from build123d import *

# Parameters (mm, degrees)
SKETCH7_W           = 90
SKETCH7_H           = 65
BOSS_EXTRUDE2_DEPTH = 65
SKETCH10_W          = 86
SKETCH10_H          = 61
CUT_EXTRUDE2_DEPTH  = 62
SKETCH12_R          = 15
CUT_EXTRUDE3_DEPTH  = 91
SKETCH13_R          = 21
SKETCH13_R_2        = 3
CUT_EXTRUDE4_DEPTH  = 2
SKETCH14_W          = 7
SKETCH14_H          = 17.962946586
CUT_EXTRUDE5_DEPTH  = 5
SKETCH15_W          = 84
SKETCH15_H          = 26.21557427
CUT_EXTRUDE6_DEPTH  = 5
SKETCH17_W          = 30
SKETCH17_H          = 32.5
BOSS_EXTRUDE3_DEPTH = 15
SKETCH18_W          = 12.726486876
SKETCH18_H          = 30.948281703
CUT_EXTRUDE7_DEPTH  = 91
SKETCH20_W          = 24.28117476
SKETCH20_H          = 6.721130416
BOSS_EXTRUDE4_DEPTH = 10
SKETCH21_W          = 21.308601662
SKETCH21_H          = 6.528068718
CUT_EXTRUDE9_DEPTH  = 52.082060801
BOSS_EXTRUDE5_DEPTH = 5
SKETCH24_R          = 1.516132664
SKETCH24_R_2        = 1.46792115
CUT_EXTRUDE10_DEPTH = 3
SKETCH25_R          = 2.5
CUT_EXTRUDE11_DEPTH = 1


with BuildPart() as part:
    # Sketch7 → Boss-Extrude2 (new body)
    with BuildSketch(Plane(origin=(0, 0, 0), x_dir=(1, 0, 0), z_dir=(0, 1, 0))):
        Rectangle(SKETCH7_W, SKETCH7_H)
    extrude(amount=-BOSS_EXTRUDE2_DEPTH)

    # Sketch10 → Cut-Extrude2 (cut)
    with BuildSketch(Plane(origin=(0, 0, 0), x_dir=(1, 0, 0), z_dir=(0, 1, 0))):
        Rectangle(SKETCH10_W, SKETCH10_H)
    extrude(amount=-CUT_EXTRUDE2_DEPTH, mode=Mode.SUBTRACT)

    # Sketch12 → Cut-Extrude3 (cut, through all)
    with BuildSketch(Plane.ZY.offset(45)):
        with Locations((0, -32.5)):
            Circle(SKETCH12_R)
    extrude(amount=-CUT_EXTRUDE3_DEPTH, mode=Mode.SUBTRACT)

    # Sketch13 → Cut-Extrude4 (cut)
    with BuildSketch(Plane.XY.offset(32.5)):
        with Locations((0, -32.5)):
            Circle(SKETCH13_R)
        with Locations((-38.356194479, -9.309094371)):
            Circle(SKETCH13_R_2)
        with Locations((-38.356194479, -19.309094371)):
            Circle(SKETCH13_R_2)
        with Locations((-38.356194479, -29.309094371)):
            Circle(SKETCH13_R_2)
        with Locations((-38.356194479, -39.309094371)):
            Circle(SKETCH13_R_2)
        with Locations((36.896991428, -19.309094371)):
            Circle(SKETCH13_R_2)
        with Locations((36.896991428, -29.309094371)):
            Circle(SKETCH13_R_2)
    extrude(amount=-CUT_EXTRUDE4_DEPTH, mode=Mode.SUBTRACT)

    # Sketch14 → Cut-Extrude5 (cut)
    with BuildSketch(Plane(origin=(45, 0, 0), x_dir=(0, 0, -1), z_dir=(1, 0, 0))):
        with Locations((26, -52.018526707)):
            Rectangle(SKETCH14_W, SKETCH14_H)
    extrude(amount=-CUT_EXTRUDE5_DEPTH, mode=Mode.SUBTRACT)

    # Sketch15 → Cut-Extrude6 (cut)
    with BuildSketch(Plane.XZ.offset(65)):
        with Locations((0, -13.392212865)):
            Rectangle(SKETCH15_W, SKETCH15_H)
    extrude(amount=-CUT_EXTRUDE6_DEPTH, mode=Mode.SUBTRACT)

    # Sketch17 → Boss-Extrude3 (add)
    with BuildSketch(Plane(origin=(0, 0, -32.5), x_dir=(-1, 0, 0), z_dir=(0, 0, -1))):
        with Locations((-30, -16.25)):
            Rectangle(SKETCH17_W, SKETCH17_H)
        with Locations((30, -16.25)):
            Rectangle(SKETCH17_W, SKETCH17_H)
    extrude(amount=BOSS_EXTRUDE3_DEPTH)

    # Sketch18 → Cut-Extrude7 (cut, through all)
    with BuildSketch(Plane(origin=(45, 0, 0), x_dir=(0, 0, -1), z_dir=(1, 0, 0))):
        with Locations((40.003797932, -17.025859149)):
            Rectangle(SKETCH18_W, SKETCH18_H)
    extrude(amount=-CUT_EXTRUDE7_DEPTH, mode=Mode.SUBTRACT)

    # Sketch20 → Boss-Extrude4 (add)
    with BuildSketch(Plane(origin=(0, 0, -32.5), x_dir=(-1, 0, 0), z_dir=(0, 0, -1))):
        with Locations((0, -57.278504407)):
            Rectangle(SKETCH20_W, SKETCH20_H)
        with Locations((0, -17.278504407)):
            Rectangle(SKETCH20_W, SKETCH20_H)
    extrude(amount=BOSS_EXTRUDE4_DEPTH)

    # Sketch21 → Cut-Extrude9 (cut, through all)
    with BuildSketch(Plane(origin=(0, -13.917939199, 0), x_dir=(1, 0, 0), z_dir=(0, 1, 0))):
        with Locations((-0.070940944, 37.501061987)):
            Rectangle(SKETCH21_W, SKETCH21_H)
    extrude(amount=-CUT_EXTRUDE9_DEPTH, mode=Mode.SUBTRACT)

    # Sketch23 → Boss-Extrude5 (add)
    with BuildSketch(Plane(origin=(0, 0, 0), x_dir=(1, 0, 0), z_dir=(0, 1, 0))):
        with BuildLine():
            Line((43, -28.521055724), (43, -30.5))
            Line((43, -30.5), (41.021055724, -30.5))
            ThreePointArc((41.021055724, -30.5), (41.600675083, -29.100675083), (43, -28.521055724))
        make_face()
        with BuildLine():
            Line((-43, -28.521055724), (-43, -30.5))
            Line((-43, -30.5), (-41.021055724, -30.5))
            ThreePointArc((-41.021055724, -30.5), (-41.600675083, -29.100675083), (-43, -28.521055724))
        make_face()
    extrude(amount=-BOSS_EXTRUDE5_DEPTH)

    # Sketch24 → Cut-Extrude10 (cut)
    with BuildSketch(Plane(origin=(0, 0, 0), x_dir=(1, 0, 0), z_dir=(0, 1, 0))):
        with Locations((-43, -30.5)):
            Circle(SKETCH24_R)
        with Locations((43, -30.5)):
            Circle(SKETCH24_R_2)
    extrude(amount=-CUT_EXTRUDE10_DEPTH, mode=Mode.SUBTRACT)

    # Sketch25 → Cut-Extrude11 (cut)
    with BuildSketch(Plane.XZ.offset(65)):
        with Locations((0, -28.5)):
            Circle(SKETCH25_R)
    extrude(amount=-CUT_EXTRUDE11_DEPTH, mode=Mode.SUBTRACT)


solid = part.part
Could you check a few things on this model? Use its own coordinates, in mm. A direction names the side the tool comes from. Give positions to 0.01 mm unless a question says otherwise; leave off trailing zeros. Order: outer loops, then holes, each group sorted by start corner. A loop starts at its lowest first (then second) coordinate and runs counter-clockwise, first axis right, second up. Notation, with made-up numbers: (-36.75, 67.25) - (-11.75, 67.25) arc R29 ccw to (-11.75, 94.25) - close; hole circle Ø9 at (7.25, 71.25). An arc over 180 degrees is marked (long way). Return JSON: item names as keys, results as strings. Group by question number.
Q1. Suppose I cut it at B-B, the plane z = -18.5. Please give me the cut outline in (x, y).
Q2. Suppose I cut it at A-A, the plane x = 0. State how many separate pieces and enclosed holes the cut face has, and give its area (3 significant figures).
Q3. Thinking about a two-plate mould opening in Y: for faces 1 (the face through (9.69, -51.13, 31.51)), 2 (the face through (45, -19, -7)), 3 (the face through (0, 0, -31)), which applies, pulls with the +Y half, pulls with the -Y half, needs draft (parallel to the pull), parting line crosses it, or undercut?
Q4. Which directions (+Z, -Z, +X, -X, +Y, -Y) give clear straight access to the entire face, cutting with the end or side of a thin tool? Please do faces 4 (the face through (0, -17, -34.237)), 5 (the face through (-43, -3, 30)), 6 (the face through (-30, -17, -46.367)), 7 (the face through (-36.97, -41.97, 31.51)).
Q5. Will these pins go through, and if not, where does the flat tip stop? pin 1 Ø11 at (x, z) = (-3.5, -40) entering from -Y; pin 2 Ø10 at (x, y) = (3.5, -34) entering from -Z; pin 3 Ø1 at (x, y) = (-8.5, -25.5) entering from +Z.
Q6. Suppose I cut it at D-D, the plane y = -56.5. Please give me the cut outline in (x, z).
Q7. Suppose I cut it at C-C, the plane x = 26.5. Please give me the cut outline in (y, z).
Q8. Please list where these lines run through material, in increasing order: line 1 along Z through (x, y) = (19, -14.5); line 2 along X through (y, z) = (-6, -11); line 3 along Z through (x, y) = (28.5, -38). Write a range as [from, to].
Resolved:
{
 "1": {"outline": "(-45, -65) - (-42, -65) - (-42, -62) - (-43, -62) - (-43, 0) - (-45, 0) - close; (42, -65) - (45, -65) - (45, 0) - (43, 0) - (43, -62) - (42, -62) - close"},
 "2": {"separate pieces": "5", "enclosed holes": "0", "area": "323 mm2"},
 "3": {"face 1": "undercut", "face 2": "needs draft", "face 3": "pulls with the +Y half"},
 "4": {"face 4": "+Y, -Y", "face 5": "+Y", "face 6": "+X, -X, -Y", "face 7": "+Z"},
 "5": {"pin 1": "stops at y = -60.64", "pin 2": "stops at z = -32.5", "pin 3": "stops at z = -30.5"},
 "6": {"outline": "(-45, -32.5) - (-12.14, -32.5) - (-12.14, -42.5) - (12.14, -42.5) - (12.14, -32.5) - (45, -32.5) - (45, -29.5) - (43, -29.5) - (43, -30.5) - (-43, -30.5) - (-43, 30.5) - (43, 30.5) - (43, -22.5) - (45, -22.5) - (45, 32.5) - (-45, 32.5) - close; hole (-10.73, -40.77) - (10.58, -40.77) - (10.58, -34.24) - (-10.73, -34.24) - close"},
 "7": {"outline": "(-65, -32.5) - (-32.5, -32.5) - (-32.5, -33.64) - (-1.55, -33.64) - (-1.55, -46.37) - (-32.5, -46.37) - (-32.5, -47.5) - (0, -47.5) - (0, -30.5) - (-62, -30.5) - (-62, -26.5) - (-65, -26.5) - close; (-65, -0.28) - (-62, -0.28) - (-62, 30.5) - (0, 30.5) - (0, 32.5) - (-65, 32.5) - close"},
 "8": {"line 1": "z = [-47.5, -46.37], [-33.64, -30.5], [30.5, 32.5]", "line 2": "x = [-45, -43], [43, 45]", "line 3": "z = [-32.5, -30.5], [30.5, 32.5]"}
}
